from build123d import *

# Parameters (mm, degrees)
SKETCH1_R           = 5.08
BOSS_EXTRUDE1_DEPTH = 3.175
CUT_EXTRUDE1_DEPTH  = 1.5875


with BuildPart() as part:
    # Sketch1 → Boss-Extrude1 (new body)
    with BuildSketch(Plane.XY):
        with BuildLine():
            Line((1.654255886, 83.456903623), (355.928440518, 83.456903623))
            ThreePointArc((355.928440518, 83.456903623), (375.685003985, 75.273467089), (383.868440518, 55.516903623))
            Line((383.868440518, 55.516903623), (383.868440518, 19.399703332))
            ThreePointArc((383.868440518, 19.399703332), (375.685003985, -0.356860135), (355.928440518, -8.540296668))
            Line((355.928440518, -8.540296668), (1.654255886, -8.540296668))
            ThreePointArc((1.654255886, -8.540296668), (-18.10230758, -0.356860135), (-26.285744114, 19.399703332))
            Line((-26.285744114, 19.399703332), (-26.285744114, 55.516903623))
            ThreePointArc((-26.285744114, 55.516903623), (-18.10230758, 75.273467089), (1.654255886, 83.456903623))
        make_face()
        with Locations((-17.266410752, 37.458303477)):
            Circle(SKETCH1_R, mode=Mode.SUBTRACT)
    extrude(amount=BOSS_EXTRUDE1_DEPTH)

    # Sketch2 → Cut-Extrude1 (cut)
    # profile 1 of 4: a face of its own
    with BuildSketch(Plane.XY.offset(3.175)):
        with BuildLine():
            add(Edge.make_bspline(
                [(80.116160991, 75.979814241), (80.572945846, 75.96838805), (81.464390071, 75.946089122), (82.761585994, 75.753265531), (83.980876738, 75.440347312), (85.118214528, 75.001140575), (86.167411339, 74.432836909), (87.120305277, 73.724053119), (88.006862222, 72.910504162), (88.781572714, 71.965880548), (89.463729353, 70.949833691), (89.998399018, 69.858693237), (90.395196355, 68.718158749), (90.649199151, 67.529264566), (90.751859695, 66.288698388), (90.742663347, 64.996679474), (90.564024557, 63.652201513), (90.342563176, 62.756325839), (90.228978328, 62.296842105)],
                knots=[0, 0, 0, 0, 1.092991326, 2.13304096, 3.131445324, 4.100957639, 5.0444535, 5.97821715, 6.937276196, 7.91745169, 8.895536054, 9.86089696, 10.817407172, 11.77982689, 12.762650102, 13.791815242, 14.867448903, 16, 16, 16, 16], degree=3))
            Line((90.228978328, 62.296842105), (73.494860681, -0.110092879))
            Line((73.494860681, -0.110092879), (51.963839009, -0.110092879))
            Line((51.963839009, -0.110092879), (67.408297214, 57.405572755))
            Line((67.408297214, 57.405572755), (42.07120743, 57.405572755))
            Line((42.07120743, 57.405572755), (28.482600619, 43.911331269))
            Line((28.482600619, 43.911331269), (28.37250774, 44.021424149))
            Line((28.37250774, 44.021424149), (16.529659443, -0.110092879))
            Line((16.529659443, -0.110092879), (-5.001362229, -0.110092879))
            Line((-5.001362229, -0.110092879), (15.444458204, 75.979814241))
            Line((15.444458204, 75.979814241), (36.959752322, 76.089907121))
            Line((36.959752322, 76.089907121), (30.008173375, 50.328173375))
            Line((30.008173375, 50.328173375), (51.098823529, 71.198637771))
            add(Edge.make_bspline(
                [(51.098823529, 71.198637771), (51.496763688, 71.577188987), (52.27625468, 72.318700635), (53.521895338, 73.303761259), (54.816419285, 74.114204336), (56.128007139, 74.809775832), (57.488939848, 75.322665393), (58.877070061, 75.707773792), (60.302751754, 75.930755526), (61.263328154, 75.963398777), (61.746377709, 75.979814241)],
                knots=[0, 0, 0, 0, 1.099200487, 2.15312996, 3.172151549, 4.153175518, 5.119892887, 6.077164679, 7.033054793, 8, 8, 8, 8], degree=3))
            Line((61.746377709, 75.979814241), (80.116160991, 75.979814241))
        make_face()
    # profile 2 of 4: a face of its own
    with BuildSketch(Plane.XY.offset(3.175)):
        with BuildLine():
            Line((118.145386997, 57.61003096), (116.950092879, 56.414736842))
            Line((116.950092879, 56.414736842), (110.533250774, 32.39876161))
            Line((110.533250774, 32.39876161), (129.123219814, 50.878637771))
            Line((129.123219814, 50.878637771), (161.521981424, 50.878637771))
            Line((161.521981424, 50.878637771), (157.071083591, 34.238885449))
            Line((157.071083591, 34.238885449), (117.390464396, 34.238885449))
            Line((117.390464396, 34.238885449), (108.693126935, 25.651640867))
            Line((108.693126935, 25.651640867), (106.837275542, 18.58996904))
            Line((106.837275542, 18.58996904), (151.849535604, 18.58996904))
            Line((151.849535604, 18.58996904), (165.438142415, 32.068482972))
            Line((165.438142415, 32.068482972), (168.473560372, 30.322724458))
            Line((168.473560372, 30.322724458), (142.821919505, 4.781176471))
            add(Edge.make_bspline(
                [(142.821919505, 4.781176471), (142.42558897, 4.40563779), (141.648400195, 3.669221032), (140.378629909, 2.72983858), (139.086443259, 1.922007685), (137.759547175, 1.249330178), (136.38410853, 0.749693532), (134.97817596, 0.386207664), (133.534361605, 0.157196007), (132.557907008, 0.125909425), (132.064272446, 0.110092879)],
                knots=[0, 0, 0, 0, 1.087710149, 2.132957327, 3.142311131, 4.123953504, 5.092881289, 6.053713067, 7.016078678, 8, 8, 8, 8], degree=3))
            Line((132.064272446, 0.110092879), (94.019318885, 0.110092879))
            add(Edge.make_bspline(
                [(94.019318885, 0.110092879), (93.562533058, 0.121495697), (92.671086936, 0.143749009), (91.373904534, 0.336897705), (90.159302422, 0.647440779), (89.030743975, 1.086514673), (88.001085474, 1.669343073), (87.027661194, 2.337531495), (86.162052775, 3.167267257), (85.395324382, 4.11011912), (84.737343068, 5.138224272), (84.219465728, 6.234858978), (83.812687134, 7.369301457), (83.586471856, 8.568042434), (83.471463009, 9.811604079), (83.509196493, 11.108834081), (83.679845331, 12.453440135), (83.902432286, 13.3493112), (84.016594427, 13.80879257)],
                knots=[0, 0, 0, 0, 1.094945795, 2.136855229, 3.137044923, 4.096584279, 5.030749513, 5.969051044, 6.920650617, 7.894578144, 8.878114772, 9.839711021, 10.797931648, 11.759527897, 12.756631189, 13.787866602, 14.865423694, 16, 16, 16, 16], degree=3))
            Line((84.016594427, 13.80879257), (88.042848297, 28.922972136))
            add(Edge.make_bspline(
                [(88.042848297, 28.922972136), (88.304583021, 29.762249011), (88.829432829, 31.445229009), (90.10811721, 33.789754209), (91.637210285, 36.050838621), (92.922716932, 37.371021477), (93.578947368, 38.04495356)],
                knots=[0, 0, 0, 0, 0.975136166, 1.955415087, 2.956272335, 4, 4, 4, 4], degree=3))
            Line((93.578947368, 38.04495356), (125.647430341, 69.798885449))
            add(Edge.make_bspline(
                [(125.647430341, 69.798885449), (126.173613681, 70.301463912), (127.199856843, 71.281669234), (128.852623455, 72.559024637), (130.536996878, 73.662817435), (132.286478981, 74.531301715), (134.063374504, 75.247349918), (135.898052148, 75.724007994), (137.772865678, 76.040497331), (139.040772571, 76.073408073), (139.676408669, 76.089907121)],
                knots=[0, 0, 0, 0, 1.104987577, 2.155115633, 3.169368792, 4.159784375, 5.118388166, 6.074904324, 7.034897349, 8, 8, 8, 8], degree=3))
            Line((139.676408669, 76.089907121), (183.697832817, 76.089907121))
            Line((183.697832817, 76.089907121), (178.696470588, 57.61003096))
            Line((178.696470588, 57.61003096), (118.145386997, 57.61003096))
        make_face()
    # profile 3 of 4: a face of its own
    with BuildSketch(Plane.XY.offset(3.175)):
        Polygon((252.002600619, 76.089907121), (273.517894737, 76.089907121), (253.087801858, 0.110092879), (231.556780186, -0.110092879), (240.254117647, 32.288668731), (206.675789474, 32.288668731), (198.088544892, 23.701424149), (191.671702786, 0.110092879), (170.140681115, -0.110092879), (190.586501548, 76.089907121), (212.101795666, 76.089907121), (199.818575851, 30.322724458), (218.518637771, 48.912693498), (244.720743034, 48.912693498), align=None)
    # profile 4 of 4: a face of its own
    with BuildSketch(Plane.XY.offset(3.175)):
        with BuildLine():
            Line((319.631083591, 76.089907121), (364.423157895, 76.089907121))
            Line((364.423157895, 76.089907121), (343.647058824, 0.110092879))
            Line((343.647058824, 0.110092879), (322.131764706, 0.110092879))
            Line((322.131764706, 0.110092879), (327.777956656, 20.870464396))
            Line((327.777956656, 20.870464396), (296.149845201, 20.870464396))
            Line((296.149845201, 20.870464396), (284.731640867, 9.562352941))
            Line((284.731640867, 9.562352941), (282.230959752, 0.110092879))
            Line((282.230959752, 0.110092879), (260.715665635, 0.110092879))
            Line((260.715665635, 0.110092879), (267.667244582, 25.981919505))
            add(Edge.make_bspline(
                [(267.667244582, 25.981919505), (267.86289602, 26.645371072), (268.253866848, 27.971148241), (268.999777356, 29.910929371), (269.877436893, 31.800461991), (270.912218434, 33.634395292), (272.071806246, 35.421190898), (273.36391227, 37.159516171), (274.805405218, 38.829815678), (275.840128897, 39.895431078), (276.364582043, 40.435541796)],
                knots=[0, 0, 0, 0, 0.972188851, 1.942727767, 2.918792729, 3.89888478, 4.900660299, 5.911935627, 6.941657613, 8, 8, 8, 8], degree=3))
            Line((276.364582043, 40.435541796), (306.372755418, 70.223529412))
            add(Edge.make_bspline(
                [(306.372755418, 70.223529412), (306.868599043, 70.68811599), (307.842110474, 71.600259095), (309.403215924, 72.799594193), (311.01411719, 73.806711452), (312.651676458, 74.649150324), (314.336608539, 75.305189439), (316.067863306, 75.757242357), (317.839849704, 76.032176586), (319.032476302, 76.07061432), (319.631083591, 76.089907121)],
                knots=[0, 0, 0, 0, 1.09520327, 2.15026038, 3.168190723, 4.15492977, 5.115689715, 6.0773418, 7.034972711, 8, 8, 8, 8], degree=3))
        make_face()
        with BuildLine():
            Line((332.134489164, 37.400123839), (337.560495356, 57.61003096))
            Line((337.560495356, 57.61003096), (298.540433437, 57.61003096))
            Line((298.540433437, 57.61003096), (297.345139319, 56.414736842))
            Line((297.345139319, 56.414736842), (286.58749226, 16.199380805))
            Line((286.58749226, 16.199380805), (304.076532508, 33.483962848))
            add(Edge.make_bspline(
                [(304.076532508, 33.483962848), (304.401991303, 33.793484328), (305.041456362, 34.401635574), (306.065728499, 35.204466573), (307.125276195, 35.892296283), (308.222062479, 36.433077589), (309.339430868, 36.874999281), (310.492804301, 37.163848907), (311.676386408, 37.365984392), (312.479426341, 37.388687169), (312.883962848, 37.400123839)],
                knots=[0, 0, 0, 0, 1.088018936, 2.137751703, 3.149265309, 4.143636785, 5.096896491, 6.055307392, 7.020348651, 8, 8, 8, 8], degree=3))
            Line((312.883962848, 37.400123839), (332.134489164, 37.400123839))
        make_face(mode=Mode.SUBTRACT)
    extrude(amount=-CUT_EXTRUDE1_DEPTH, mode=Mode.SUBTRACT)


solid = part.part
Geometry: final body of the model. Coordinates: model frame, mm. A direction names the side the tool comes from. Give positions to 0.01 mm unless a question says otherwise; leave off trailing zeros. Order: outer loops, then holes, each group sorted by start corner. A loop starts at its lowest first (then second) coordinate and runs counter-clockwise, first axis right, second up. Notation, with made-up numbers: (13, -1.5) -> (68, -1.5) arc R38 cw to (68, 37.5) -> close; hole circle Ø6 at (84, -38). An arc over 180 degrees is marked (long way). Answer as a JSON object with one key per item and string values.
Q1. Section A-A (z = 0.85). Output: boundary loops of the cut face in (x, y).
Entries:
{"outline": "(-26.29, 19.4) arc R27.94 ccw to (1.65, -8.54) -> (355.93, -8.54) arc R27.94 ccw to (383.87, 19.4) -> (383.87, 55.52) arc R27.94 ccw to (355.93, 83.46) -> (1.65, 83.46) arc R27.94 ccw to (-26.29, 55.52) -> close; hole circle Ø10.16 at (-17.27, 37.46)"}
Q2. Material intervals for probe 1 along Y at (x, z) = (136, 2.5); probe 2 along Y at (x, z) = (191, 2.8); probe 3 along X at (y, z) = (19, 0.9), sorted ascending.
Entries:
{"probe 1": "y = -8.54 to 0.66, 18.59 to 34.24, 50.88 to 57.61, 75.72 to 83.46", "probe 2": "y = -8.54 to 0.1, 76.09 to 83.46", "probe 3": "x = -26.28 to 383.87"}
Q3. First-contact query: pin 1 (2 mm diameter, centred on x = 269, y = 7.5, fed in from +Z). Flat tip, straight axial feed; report the tip coordinate or a pass-through.
Entries:
{"pin 1": "stops at z = 1.59"}
Q4. Access query for faces 4 (the flat face through (119.7, 41.51, 2.39)), 5 (the cylindrical face through (375.467, 75.49, 1.565)). Directions: +Z, -Z, +X, -X, +Y, -Y. A direction counts if a zero-diameter tool reaches every point of the face in a straight line with its end or side. Return the directions, or none.
Entries:
{"face 4": "+Z", "face 5": "+Z, -Z, +X, +Y"}
Q5. Draft query along X for faces 1 (the cylindrical face through (-18.318, 75.055, 1.565)), 2 (the cylindrical face through (375.9, -0.14, 1.57)), 3 (the flat face through (40.41, 60.62, 2.39)). Return one class per face: released by +X, released by -X, zero draft, split by the parting line, or undercut.
Entries:
{"face 1": "released by -X", "face 2": "released by +X", "face 3": "undercut"}
